Verification items for the finished model (mm, model axes). Face numbers are marked on the shaded views. Round coordinates to 2 decimals unless told otherwise and drop trailing zeros. Loops run counter-clockwise (first coordinate to the right, second up) from the corner with the lowest first, then second, coordinate; pieces in that order, holes last. Notation, with made-up numbers: (-37.5, 60.5) -> (-27.5, 60.5) arc R20 cw to (-27.5, 70.5) -> close; hole circle Ø6 at (72, 77.5). An arc over 180 degrees is marked (long way). Use CSV: the item, a comma, the result in double quotes. Start each with the question number.
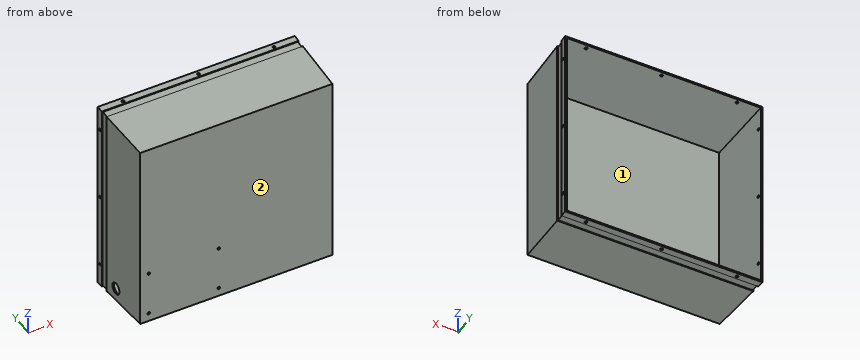
```python
from build123d import *

# Parameters (mm, degrees)
SKETCH1_W                       = 242.1
SKETCH1_H                       = 242.1
BOSS_EXTRUDE1_DEPTH             = 90
BOSS_EXTRUDE1_DRAFT             = -2
SHELL1_T                        = -2
CUT_EXTRUDE7_DEPTH              = 291.648708719
CUT_EXTRUDE8_DEPTH              = 291.648708719
M3_CLEARANCE_HOLE2_D            = 3.4
SKETCH15_R                      = 1.7
CUT_EXTRUDE9_DEPTH              = 10
SKETCH16_R                      = 1.7
CUT_EXTRUDE10_DEPTH             = 10
CUT_EXTRUDE11_DEPTH             = 198.351811614
CUT_EXTRUDE11_DEPTH_BACK        = 198.351811614
CUT_EXTRUDE12_REACH             = 292.104
SKETCH21_R                      = 7.4
CUT_EXTRUDE12_DIRECTION_2_DEPTH = 291.103764671


with BuildPart() as part:
    # Sketch1 → Boss-Extrude1 (with draft: the straight prism first)
    with BuildSketch(Plane(origin=(0, 0, 0), x_dir=(1, 0, 0), z_dir=(0, 1, 0))):
        Rectangle(SKETCH1_W, SKETCH1_H)
    extrude(amount=BOSS_EXTRUDE1_DEPTH)
    # Boss-Extrude1: the draft: its side faces are tilted about the plane it starts from
    boss_extrude1_sides = [part.faces().sort_by_distance(p)[0] for p in [
        (0, 45, 121.05),
        (121.05, 45, 0),
        (0, 45, -121.05),
        (-121.05, 45, 0),
    ]]
    draft(boss_extrude1_sides, Plane(origin=(0, 0, 0), x_dir=(1, 0, 0), z_dir=(0, 1, 0)), BOSS_EXTRUDE1_DRAFT)

    # Shell1
    shell1_openings = [part.faces().sort_by_distance(p)[0] for p in [
        (0, 90, 0),
    ]]
    offset(amount=SHELL1_T, openings=shell1_openings, kind=Kind.INTERSECTION)

    # Sketch6 → Cut-Extrude7 (cut, through all, along a direction that is not the sketch's normal)
    with BuildSketch(Plane(origin=(0, -4.222010573, 120.902564142), x_dir=(1, 0, 0), z_dir=(0, -0.03489949670250105, 0.9993908270190958))):
        Polygon((-123.843874287, 84.279443063), (-123.49509166, 74.28552738), (-122.494482858, 74.28552738), (-122.843265485, 84.279443063), align=None)
    cut_extrude7 = extrude(amount=-CUT_EXTRUDE7_DEPTH, dir=(0, 0, 1), mode=Mode.SUBTRACT)

    # Sketch7 → Cut-Extrude8 (cut, through all, along a direction that is not the sketch's normal)
    with BuildSketch(Plane(origin=(-120.902564142, -4.222010573, 0), x_dir=(0, 0, 1), z_dir=(-0.9993908270190958, -0.03489949670250105, 0))):
        Polygon((123.845093004, 84.279443063), (122.845093004, 84.279443063), (122.496310376, 74.28552738), (123.496310376, 74.28552738), align=None)
    cut_extrude8 = extrude(amount=-CUT_EXTRUDE8_DEPTH, dir=(-1, 0, 0), mode=Mode.SUBTRACT)

    # Mirror1: Cut-Extrude7 across plane
    add(cut_extrude7.mirror(Plane(origin=(0, 0, 0), x_dir=(0, 0, 1), z_dir=(1, 0, 0))), mode=Mode.SUBTRACT)

    # Mirror2: Cut-Extrude8 across plane
    add(cut_extrude8.mirror(Plane.XY), mode=Mode.SUBTRACT)

    # M3 Clearance Hole2 (through all)
    with Locations(Plane(origin=(0, 2, 0), x_dir=(1, 0, 0), z_dir=(0, 1, 0))):
        with Locations((-110.11862245, 54.11862245), (-110.11862245, 110.11862245), (-22.11862245, 110.11862245), (-22.11862245, 54.11862245)):
            Hole(M3_CLEARANCE_HOLE2_D / 2)

    # Sketch15 → Cut-Extrude9 (cut)
    with BuildSketch(Plane(origin=(0, -4.222010573, 120.902564142), x_dir=(1, 0, 0), z_dir=(0, -0.03489949670250105, 0.9993908270190958))):
        with Locations(Location((0, 88.279443063, 0), (0, 0, 270))):
            Circle(SKETCH15_R)
        with Locations(Location((-95, 88.279443063, 0), (0, 0, 270))):
            Circle(SKETCH15_R)
        with Locations(Location((95, 88.279443063, 0), (0, 0, 270))):
            Circle(SKETCH15_R)
    cut_extrude9 = extrude(amount=-CUT_EXTRUDE9_DEPTH, mode=Mode.SUBTRACT)

    # Mirror3: Cut-Extrude9 across plane
    add(cut_extrude9.mirror(Plane.XY), mode=Mode.SUBTRACT)

    # Sketch16 → Cut-Extrude10 (cut)
    with BuildSketch(Plane(origin=(-120.902564142, -4.222010573, 0), x_dir=(0, 0, 1), z_dir=(-0.9993908270190958, -0.03489949670250105, 0))):
        with Locations(Location((0, 88.279443063, 0), (0, 0, 270))):
            Circle(SKETCH16_R)
        with Locations(Location((95, 88.279443063, 0), (0, 0, 270))):
            Circle(SKETCH16_R)
        with Locations(Location((-95, 88.279443063, 0), (0, 0, 270))):
            Circle(SKETCH16_R)
    cut_extrude10 = extrude(amount=-CUT_EXTRUDE10_DEPTH, mode=Mode.SUBTRACT)

    # Mirror4: Cut-Extrude10 across plane
    add(cut_extrude10.mirror(Plane(origin=(0, 0, 0), x_dir=(0, 0, 1), z_dir=(1, 0, 0))), mode=Mode.SUBTRACT)

    # Sketch18 → Cut-Extrude11 (cut, two sides: drawn at the far end of the back side and taken through both)
    with BuildSketch(Plane.XY.offset(-CUT_EXTRUDE11_DEPTH_BACK)):
        Polygon((-124.192869254, 90), (-124.157948485, 89), (124.157948485, 89), (124.192869254, 90), align=None)
    extrude(amount=CUT_EXTRUDE11_DEPTH + CUT_EXTRUDE11_DEPTH_BACK, mode=Mode.SUBTRACT)

    # Sketch21 → Cut-Extrude12 (cut, up to next)
    with BuildSketch(Plane(origin=(-120.902564142, -4.222010573, 0), x_dir=(0, 0, 1), z_dir=(-0.9993908270190958, -0.03489949670250105, 0)), mode=Mode.PRIVATE) as cut_extrude12_sk1:
        with Locations(Location((-106.300517026, 54.932485221, 0), (0, 0, 270))):
            Circle(SKETCH21_R)
    cut_extrude12_tool1 = extrude(cut_extrude12_sk1.sketch, amount=-CUT_EXTRUDE12_REACH, mode=Mode.PRIVATE) & part.part
    add(cut_extrude12_tool1.solids().sort_by_distance((-122.81968, 50.677011, -106.300517))[0], mode=Mode.SUBTRACT)

    # Sketch21 → Cut-Extrude12 direction 2 (cut)
    with BuildSketch(Plane(origin=(-120.902564142, -4.222010573, 0), x_dir=(0, 0, 1), z_dir=(-0.9993908270190958, -0.03489949670250105, 0))):
        with Locations(Location((-106.300517026, 54.932485221, 0), (0, 0, 270))):
            Circle(SKETCH21_R)
    extrude(amount=CUT_EXTRUDE12_DIRECTION_2_DEPTH, mode=Mode.SUBTRACT)


solid = part.part
```
Q1. Cross-section at D-D (y = 75.5). Record the boundary of the cut face in (x, z).
Q2. Cross-section at C-C (z = -31). Record the boundary of the cut face in (x, y).
Q3. Release check for a two-part mould opening along Z. For the marked faces 1 and 2 record: +Z half, -Z half, draft (parallel to the pull), parting line (faces both ways), or undercut.
Q4. Cross-section at B-B (y = 6). Record the boundary of the cut face in (x, z), and give its area (3 significant figures).
Q5. Depth check by flat-ended pin: pin 1 Ø3 at (x, z) = (29, 61) entering from +Y; pin 2 Ø1.5 at (x, y) = (32, 79.5) entering from -Z; pin 3 Ø1.5 at (x, y) = (-51.5, 18) entering from -Z; pin 4 Ø2 at (x, z) = (-110.12, -54.12) entering from +Y. Enter the tip coordinate at first touch or a pass-through.
Q6. Thickness scan on L1, parallel to Y at x = -19, z = 10; L2, parallel to Z at x = -1, y = 82; L3, parallel to X at y = 77.5, z = -75.5. Record the ranges inside material, lowest first. Write a range as from..to.
Q7. Cross-section at A-A (x = -79). Record the boundary of the cut face in (y, z).
Answer list:
1,outline,"(-122.69, -122.69) -> (122.69, -122.69) -> (122.69, 122.69) -> (-122.69, 122.69) -> close; hole (-121.69, -121.69) -> (121.69, -121.69) -> (121.69, 121.69) -> (-121.69, 121.69) -> close"
2,outline,"(-124.16, 89) -> (-123.84, 80.01) -> (-122.84, 80.01) -> (-122.49, 70.02) -> (-123.5, 70.02) -> (-121.05, 0) -> (121.05, 0) -> (123.5, 70.02) -> (122.49, 70.02) -> (122.84, 80.01) -> (123.84, 80.01) -> (124.16, 89) -> (122.16, 89) -> (119.12, 2) -> (-119.12, 2) -> (-122.16, 89) -> close"
3,face 1,"undercut"
3,face 2,"draft"
4,outline,"(-121.26, -121.26) -> (121.26, -121.26) -> (121.26, 121.26) -> (-121.26, 121.26) -> close; hole (-119.26, -119.26) -> (119.26, -119.26) -> (119.26, 119.26) -> (-119.26, 119.26) -> close"
4,area,"1,930 mm2"
5,pin 1,"stops at y = 2"
5,pin 2,"stops at z = -123.85"
5,pin 3,"stops at z = -121.7"
5,pin 4,"passes through"
6,L1,"y = 0..2"
6,L2,"z = -123.91..-121.91, 121.91..123.91"
6,L3,"x = -122.76..-121.76, 121.76..122.76"
7,outline,"(0, -121.05) -> (70.02, -123.5) -> (70.02, -122.5) -> (80.01, -122.85) -> (80.01, -123.84) -> (89, -124.16) -> (89, -122.16) -> (2, -119.12) -> (2, 119.12) -> (89, 122.16) -> (89, 124.16) -> (80.01, 123.84) -> (80.01, 122.85) -> (70.02, 122.5) -> (70.02, 123.5) -> (0, 121.05) -> close"
